from build123d import *

# Parameters (mm, degrees)
CROQUIS2_W                   = 90
CROQUIS2_H                   = 120
SALIENTE_EXTRUIR1_DEPTH      = 20
VACIADO1_T                   = -2
REDONDEO1_R                  = 10
CROQUIS3_R                   = 1.55
CORTAR_EXTRUIR1_DEPTH        = 20
CROQUIS4_R                   = 2.5
CROQUIS4_R_2                 = 1.15
SALIENTE_EXTRUIR2_DEPTH      = 9
CROQUIS5_W                   = 16
CROQUIS5_H                   = 9
CORTAR_EXTRUIR2_DEPTH        = 2
REDONDEO2_R                  = 1
SALIENTE_EXTRUIR3_DEPTH      = 1
GANCHO_START                 = 41
GANCHO_DE_MOSQUET_N1_DEPTH   = 2
GANCHO_START_2               = -42.549292451
GANCHO_DE_MOSQUET_N1_2_DEPTH = 4.628893351
GANCHO_START_3               = 43
GANCHO_DE_MOSQUET_N1_3_DEPTH = 3
GANCHO_DE_MOSQUET_N1_4_DEPTH = 2
SIMETR_A2_START              = 41
SIMETR_A2_COPY_1_DEPTH       = 2
SIMETR_A2_START_2            = -42.549292451
SIMETR_A2_COPY_2_DEPTH       = 4.628893351
SIMETR_A2_START_3            = 43
SIMETR_A2_COPY_3_DEPTH       = 3
SIMETR_A2_COPY_4_DEPTH       = 2


with BuildPart() as part:
    # Croquis2 → Saliente-Extruir1 (new body)
    with BuildSketch(Plane(origin=(0, 0, 0), x_dir=(1, 0, 0), z_dir=(0, 1, 0))):
        Rectangle(CROQUIS2_W, CROQUIS2_H)
    extrude(amount=SALIENTE_EXTRUIR1_DEPTH)

    # Vaciado1
    vaciado1_openings = [part.faces().sort_by_distance(p)[0] for p in [
        (0, 20, 0),
    ]]
    offset(amount=VACIADO1_T, openings=vaciado1_openings, kind=Kind.INTERSECTION)

    # Redondeo1
    redondeo1_edges = [part.edges().sort_by_distance(p)[0] for p in [
        (-43, 11, -58),
        (-43, 11, 58),
        (43, 11, 58),
        (43, 11, -58),
        (-45, 10, -60),
        (45, 10, -60),
        (45, 10, 60),
        (-45, 10, 60),
    ]]
    fillet(redondeo1_edges, radius=REDONDEO1_R)

    # Croquis3 → Cortar-Extruir1 (cut)
    with BuildSketch(Plane(origin=(0, 2, 0), x_dir=(1, 0, 0), z_dir=(0, 1, 0))):
        with Locations(Location((0, -39.225, 0), (0, 0, 270))):
            Circle(CROQUIS3_R)
        with Locations(Location((0, -19.375, 0), (0, 0, 270))):
            Circle(CROQUIS3_R)
    extrude(amount=-CORTAR_EXTRUIR1_DEPTH, mode=Mode.SUBTRACT)

    # Croquis4 → Saliente-Extruir2 (add)
    # profile 1 of 4: a face of its own
    with BuildSketch(Plane(origin=(0, 2, 0), x_dir=(1, 0, 0), z_dir=(0, 1, 0))):
        with Locations(Location((-31.9, 51.355578, 0), (0, 0, 90))):
            Circle(CROQUIS4_R)
        with Locations(Location((-31.9, 51.355578, 0), (0, 0, 270))):
            Circle(CROQUIS4_R_2, mode=Mode.SUBTRACT)
    # profile 2 of 4: a face of its own
    with BuildSketch(Plane(origin=(0, 2, 0), x_dir=(1, 0, 0), z_dir=(0, 1, 0))):
        with Locations(Location((32.5, 51.355578, 0), (0, 0, 90))):
            Circle(CROQUIS4_R)
        with Locations(Location((32.5, 51.355578, 0), (0, 0, 270))):
            Circle(CROQUIS4_R_2, mode=Mode.SUBTRACT)
    # profile 3 of 4: a face of its own
    with BuildSketch(Plane(origin=(0, 2, 0), x_dir=(1, 0, 0), z_dir=(0, 1, 0))):
        with Locations(Location((32.35, -0.544422, 0), (0, 0, 90))):
            Circle(CROQUIS4_R)
        with Locations(Location((32.35, -0.544422, 0), (0, 0, 270))):
            Circle(CROQUIS4_R_2, mode=Mode.SUBTRACT)
    # profile 4 of 4: a face of its own
    with BuildSketch(Plane(origin=(0, 2, 0), x_dir=(1, 0, 0), z_dir=(0, 1, 0))):
        with Locations(Location((-32.05, -0.544422, 0), (0, 0, 90))):
            Circle(CROQUIS4_R)
        with Locations(Location((-32.05, -0.544422, 0), (0, 0, 270))):
            Circle(CROQUIS4_R_2, mode=Mode.SUBTRACT)
    extrude(amount=SALIENTE_EXTRUIR2_DEPTH)

    # Croquis5 → Cortar-Extruir2 (cut)
    with BuildSketch(Plane(origin=(45, 0, 0), x_dir=(0, 0, -1), z_dir=(1, 0, 0))):
        with Locations((21, 4.5)):
            Rectangle(CROQUIS5_W, CROQUIS5_H)
    extrude(amount=-CORTAR_EXTRUIR2_DEPTH, mode=Mode.SUBTRACT)

    # Redondeo2
    redondeo2_edges = [part.edges().sort_by_distance(p)[0] for p in [
        (44, 9, -13),
        (44, 9, -29),
    ]]
    fillet(redondeo2_edges, radius=REDONDEO2_R)

    # Croquis6 → Saliente-Extruir3 (add)
    with BuildSketch(Plane(origin=(0, 2, 0), x_dir=(1, 0, 0), z_dir=(0, 1, 0))):
        Polygon((43, 29.794557256), (16.5, 29.794557256), (16.5, 12.4), (43, 12.4), (43, 11.9), (16, 11.9), (16, 30.294557256), (43, 30.294557256), align=None)
    extrude(amount=SALIENTE_EXTRUIR3_DEPTH)



with BuildPart() as body_2:
    # Gancho de mosquet_n1: read off the stored shape, not the designer's step
    # Gancho de mosquet_n1 outline → Gancho de mosquet_n1 (new body)
    with BuildSketch(Plane.YZ.offset(GANCHO_START)):
        Polygon((21, -37.9203991), (21, -42.549292451), (27, -42.234845775), (27, -38.234845775), align=None)
    gancho_de_mosquet_n1 = extrude(amount=GANCHO_DE_MOSQUET_N1_DEPTH)

    # Gancho de mosquet_n1 2 outline → Gancho de mosquet_n1 2 (add)
    with BuildSketch(Plane.XY.offset(GANCHO_START_2)):
        Polygon((43, 21), (45, 21), (43, 27), align=None)
    gancho_de_mosquet_n1_2 = extrude(amount=GANCHO_DE_MOSQUET_N1_2_DEPTH)

    # Gancho de mosquet_n1 3 outline → Gancho de mosquet_n1 3 (cut)
    with BuildSketch(Plane.YZ.offset(GANCHO_START_3)):
        Polygon((27, -42.234845775), (21, -42.549292451), (28, -42.549292451), (28, -42.182437996), align=None)
        Polygon((28, -37.9203991), (21, -37.9203991), (27, -38.234845775), (28, -38.287253554), align=None)
    gancho_de_mosquet_n1_3 = extrude(amount=GANCHO_DE_MOSQUET_N1_3_DEPTH, mode=Mode.SUBTRACT)


with BuildPart() as part_1:
    add(part.part)

    add(body_2.part)  # Gancho de mosquet_n1 4 merges body 2
    # Gancho de mosquet_n1 4 outline → Gancho de mosquet_n1 4 (add)
    with BuildSketch(Plane.YZ.offset(GANCHO_START)):
        Polygon((1, -43.597448037), (2, -43.545040258), (21, -42.549292451), (21, -37.9203991), (2, -36.924651293), (1, -36.872243514), align=None)
    gancho_de_mosquet_n1_4 = extrude(amount=GANCHO_DE_MOSQUET_N1_4_DEPTH)

    # Simetr_a1: Gancho de mosquet_n1, Gancho de mosquet_n1 2, Gancho de mosquet_n1 3, Gancho de mosquet_n1 4 across plane
    add(gancho_de_mosquet_n1.mirror(Plane.XY))
    add(gancho_de_mosquet_n1_2.mirror(Plane.XY))
    add(gancho_de_mosquet_n1_3.mirror(Plane.XY), mode=Mode.SUBTRACT)
    add(gancho_de_mosquet_n1_4.mirror(Plane.XY))

    # Simetr_a2: Gancho de mosquet_n1, Gancho de mosquet_n1 2, Gancho de mosquet_n1 3, Gancho de mosquet_n1 4 across plane
    add(gancho_de_mosquet_n1.mirror(Plane(origin=(0, 0, 0), x_dir=(0, 0, 1), z_dir=(1, 0, 0))))
    add(gancho_de_mosquet_n1_2.mirror(Plane(origin=(0, 0, 0), x_dir=(0, 0, 1), z_dir=(1, 0, 0))))
    add(gancho_de_mosquet_n1_3.mirror(Plane(origin=(0, 0, 0), x_dir=(0, 0, 1), z_dir=(1, 0, 0))), mode=Mode.SUBTRACT)
    add(gancho_de_mosquet_n1_4.mirror(Plane(origin=(0, 0, 0), x_dir=(0, 0, 1), z_dir=(1, 0, 0))))



with BuildPart() as body_2_2:
    # Simetr_a2 copy 1 sketch → Simetr_a2 copy 1 (new body)
    with BuildSketch(Plane(origin=(0, 0, 0), x_dir=(0, 1, 0), z_dir=(-1, 0, 0)).offset(SIMETR_A2_START)):
        Polygon((21, -37.9203991), (21, -42.549292451), (27, -42.234845775), (27, -38.234845775), align=None)
    extrude(amount=SIMETR_A2_COPY_1_DEPTH)

    # Simetr_a2 copy 2 sketch → Simetr_a2 copy 2 (add)
    with BuildSketch(Plane(origin=(0, 0, 0), x_dir=(-1, 0, 0), z_dir=(0, 0, -1)).offset(SIMETR_A2_START_2)):
        Polygon((43, 21), (45, 21), (43, 27), align=None)
    extrude(amount=SIMETR_A2_COPY_2_DEPTH)

    # Simetr_a2 copy 3 sketch → Simetr_a2 copy 3 (cut)
    with BuildSketch(Plane(origin=(0, 0, 0), x_dir=(0, 1, 0), z_dir=(-1, 0, 0)).offset(SIMETR_A2_START_3)):
        Polygon((27, -42.234845775), (21, -42.549292451), (28, -42.549292451), (28, -42.182437996), align=None)
        Polygon((28, -37.9203991), (21, -37.9203991), (27, -38.234845775), (28, -38.287253554), align=None)
    extrude(amount=SIMETR_A2_COPY_3_DEPTH, mode=Mode.SUBTRACT)


with BuildPart() as part_2:
    add(part_1.part)

    add(body_2_2.part)  # Simetr_a2 copy 4 merges body 2 2
    # Simetr_a2 copy 4 sketch → Simetr_a2 copy 4 (add)
    with BuildSketch(Plane(origin=(0, 0, 0), x_dir=(0, 1, 0), z_dir=(-1, 0, 0)).offset(SIMETR_A2_START)):
        Polygon((1, -43.597448037), (2, -43.545040258), (21, -42.549292451), (21, -37.9203991), (2, -36.924651293), (1, -36.872243514), align=None)
    extrude(amount=SIMETR_A2_COPY_4_DEPTH)


solid = part_2.part
The listing builds one solid part. Answer for the finished solid, in the listing's coordinates (mm). A direction names the side the tool comes from. Coordinates: 2 decimals unless noted, no trailing zeros. Loops run counter-clockwise (first coordinate to the right, second up) from the corner with the lowest first, then second, coordinate; pieces in that order, holes last. Notation, with made-up numbers: (-37.75, 88) -> (-2.75, 88) arc R18 ccw to (-2.75, 117) -> close; hole circle Ø2 at (87.25, -31.75). An arc over 180 degrees is marked (long way). Answer in a Markdown table with one row per item. Add a question column.
1. Determine the mould class of faces 1 (the cylindrical face through (-42.15, 10.14, -56.99)), 2 (the cylindrical face through (29.87, 6.44, 0.87)), 3 (the flat face through (45, 10, 1)) for opening direction X: +X half, -X half, draft (parallel to the pull), parting line (faces both ways), or undercut.
2. The part is cut by section C-C, the plane x = 22. Write down the section's boundary in (y, z).
3. For faces 4 (the cylindrical face through (-29.61, 6.44, 1.09)), 5 (the cylindrical face through (0.47, 1.01, 40.7)), determine the directions among +Z, -Z, +X, -X, +Y, -Y from which every point of the face is accessible in a straight line to the end or side of a thin tool.
4. Consider line 1 (Z direction, x = 21.5, y = 5.75); line 2 (X direction, y = 17.5, z = 0); line 3 (X direction, y = 15.5, z = 42). Determine where each line is inside the solid, lowest interval first. Write a range as [from, to].
5. The part is cut by section B-B, the plane y = 24.25. Write down the section's boundary in (x, z).
6. The part is cut by section A-A, the plane x = 0. Write down the section's boundary in (y, z) (3 decimals), then the cut area to 3 significant figures.
7. Flat-ended cylindrical pins translate along their axes: P1, Ø2, axis at x = 44, y = 5, coming from the +Z side; P2, Ø0.5, axis at x = 35.5, y = 2.5, coming from the +Z side; P3, Ø5, axis at y = 3.5, z = -22, coming from the +X side. Find the tip coordinate at first contact, or state that the pin passes through.
8. The part is cut by section D-D, the plane z = 30.5. Write down the section's boundary in (x, y).
Answer below:
| question | item | result |
|---|---|---|
| 1 | face 1 | -X half |
| 1 | face 2 | undercut |
| 1 | face 3 | +X half |
| 2 | outline | (0, -60) -> (20, -60) -> (20, -58) -> (2, -58) -> (2, -30.29) -> (3, -30.29) -> (3, -29.79) -> (2, -29.79) -> (2, -12.4) -> (3, -12.4) -> (3, -11.9) -> (2, -11.9) -> (2, 58) -> (20, 58) -> (20, 60) -> (0, 60) -> close |
| 3 | face 4 | +Y |
| 3 | face 5 | +Y, -Y |
| 4 | line 1 | [-60, -58], [58, 60] |
| 4 | line 2 | [-45, -43], [43, 45] |
| 4 | line 3 | [-45, -41], [41, 45] |
| 5 | outline | (-43.92, -42.38) -> (-41, -42.38) -> (-41, -38.09) -> (-43.92, -38.09) -> close; (-43.92, 38.09) -> (-41, 38.09) -> (-41, 42.38) -> (-43.92, 42.38) -> close; (41, -42.38) -> (43.92, -42.38) -> (43.92, -38.09) -> (41, -38.09) -> close; (41, 38.09) -> (43.92, 38.09) -> (43.92, 42.38) -> (41, 42.38) -> close |
| 6 | outline | (0, -60) -> (20, -60) -> (20, -58) -> (2, -58) -> (2, 17.825) -> (0, 17.825) -> close; (0, 20.925) -> (2, 20.925) -> (2, 37.675) -> (0, 37.675) -> close; (0, 40.775) -> (2, 40.775) -> (2, 58) -> (20, 58) -> (20, 60) -> (0, 60) -> close |
| 6 | area | 300 mm2 |
| 7 | P1 | z = 56 |
| 7 | P2 | z = 60 |
| 7 | P3 | x = 43 |
| 8 | outline | (-45, 0) -> (45, 0) -> (45, 20) -> (43, 20) -> (43, 2) -> (-43, 2) -> (-43, 20) -> (-45, 20) -> close |
